Geometry check sheet. Reference: the model listing, model coordinates, mm. Face numbers are marked on the shaded views. Coordinates: 2 decimals unless noted, no trailing zeros. Write each loop counter-clockwise with the first axis right and the second up, starting at its lowest first coordinate (ties: lowest second). Pieces come first, ordered by that corner, then holes. Notation, with made-up numbers: (19.25, 1.25) -> (47.25, 1.25) arc R6 ccw to (47.25, 7.25) -> close; hole circle Ø8 at (36, -28). An arc over 180 degrees is marked (long way). Answer in a Markdown table with one row per item. Add a question column.
Q1. Section check C-C, the plane y = 44.5. Record the boundary of the cut face in (x, z), and give its area (3 significant figures).
Q2. Gauge pin test, flat ends, axial feed: P1, Ø5, axis at y = -13, z = 12, coming from the +X side; P2, Ø1, axis at x = -21, z = 4, coming from the +Y side; P3, Ø6, axis at x = -25.5, z = 15.5, coming from the +Y side. Record the tip position at first contact, or that the pin passes through.
Q3. Section check B-B, the plane x = 42. Record the boundary of the cut face in (y, z), and give its area (3 significant figures).
Q4. Section check A-A, the plane z = 11.25. Record the boundary of the cut face in (x, y).
Q5. Thickness scan on line 1 (Y direction, x = 1.5, z = 6); line 2 (Y direction, x = -4.5, z = 16.6); line 3 (X direction, y = -4.5, z = 15.85). Record the ranges inside material, lowest first.
Q6. Section check D-D, the plane x = -7.5. Count the separate pieces of the cut face and the enclosed holes in it, and give its area (3 significant figures).
Q7. Release check for a two-part mould opening along X. For the marked faces 1, 2 and 3 record: pulls with the +X half, pulls with the -X half, needs draft (parallel to the pull), parting line crosses it, or undercut.
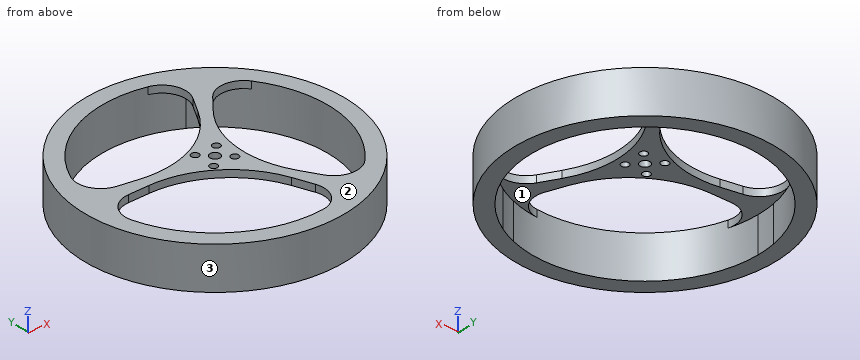
```python
from build123d import *

# Parameters (mm, degrees)
ESQUISSE1_R             = 55
BOSS_EXTRU_1_DEPTH      = 18
ESQUISSE2_R             = 2.1
ENL_V_MAT_EXTRU_1_DEPTH = 80.837334625
ENL_V_MAT_EXTRU_2_DEPTH = 80.837334625
ENL_V_MAT_EXTRU_3_DEPTH = 80.837334625
ENL_V_START             = 15
ESQUISSE8_R             = 48
ENL_V_MAT_EXTRU_4_DEPTH = 15
CONG_3_R                = 10
CONG_4_R                = 10
CONG_5_R                = 60
CONG_7_R                = 40
ESQUISSE10_R            = 1.6
ENL_V_MAT_EXTRU_9_DEPTH = 80.837334785


with BuildPart() as part:
    # Esquisse1 → Boss.-Extru.1 (new body)
    with BuildSketch(Plane.XY):
        Circle(ESQUISSE1_R)
    extrude(amount=BOSS_EXTRU_1_DEPTH)

    # Esquisse2 → Enlèv. mat.-Extru.1 (cut, through all)
    with BuildSketch(Plane.XY.offset(18)):
        Circle(ESQUISSE2_R)
    extrude(amount=-ENL_V_MAT_EXTRU_1_DEPTH, mode=Mode.SUBTRACT)

    # Esquisse3 → Enlèv. mat.-Extru.2 (cut, through all)
    with BuildSketch(Plane.XY.offset(18)):
        with BuildLine():
            ThreePointArc((-7.5, 0), (-4.301823273, -6.143640332), (2.565151075, -7.047694656))
            Line((2.565151075, -7.047694656), (16.41696688, -45.105245798))
            ThreePointArc((16.41696688, -45.105245798), (-27.531668945, -39.319298126), (-48, 0))
            Line((-48, 0), (-7.5, 0))
        make_face()
        with BuildLine():
            ThreePointArc((-47.270772145, 8.335112528), (-20.285676564, 43.502773778), (24, 41.569219382))
            Line((24, 41.569219382), (3.75, 6.495190528))
            ThreePointArc((3.75, 6.495190528), (-3.169636963, 6.797308403), (-7.386058148, 1.302361333))
            Line((-7.386058148, 1.302361333), (-47.270772145, 8.335112528))
        make_face()
        with BuildLine():
            ThreePointArc((30.853805265, 36.77013327), (47.817345508, -4.183475652), (24, -41.569219382))
            Line((24, -41.569219382), (3.75, -6.495190528))
            ThreePointArc((3.75, -6.495190528), (7.471460236, -0.653668071), (4.820907073, 5.745333323))
            Line((4.820907073, 5.745333323), (30.853805265, 36.77013327))
        make_face()
    extrude(amount=-ENL_V_MAT_EXTRU_2_DEPTH, mode=Mode.SUBTRACT)

    # Esquisse7 → Enlèv. mat.-Extru.3 (cut, through all)
    with BuildSketch(Plane.XY):
        with BuildLine():
            Line((2.565151075, -7.047694656), (-27.531668945, -39.319298126))
            Line((-27.531668945, -39.319298126), (-7.5, 0))
            ThreePointArc((-7.5, 0), (-3.331557771, -4.75795759), (2.565151075, -7.047694656))
        make_face()
        with BuildLine():
            Line((4.820907073, 5.745333323), (47.817345508, -4.183475652))
            Line((47.817345508, -4.183475652), (3.75, -6.495190528))
            ThreePointArc((3.75, -6.495190528), (5.786291029, -0.506234869), (4.820907073, 5.745333323))
        make_face()
        with BuildLine():
            Line((3.75, 6.495190528), (-20.285676564, 43.502773778))
            Line((-20.285676564, 43.502773778), (-7.386058148, 1.302361333))
            ThreePointArc((-7.386058148, 1.302361333), (-2.454733258, 5.264192459), (3.75, 6.495190528))
        make_face()
    extrude(amount=ENL_V_MAT_EXTRU_3_DEPTH, mode=Mode.SUBTRACT)

    # Esquisse8 → Enlèv. mat.-Extru.4 (cut)
    with BuildSketch(Plane.XY.offset(ENL_V_START)):
        Circle(ESQUISSE8_R)
    extrude(amount=-ENL_V_MAT_EXTRU_4_DEPTH, mode=Mode.SUBTRACT)

    # Congé3
    # the kernel refuses this fillet: 10 mm, written as the material it adds along each edge
    with BuildSketch(Plane(origin=(-47.270772145, 8.335112528, 18), x_dir=(0.3028483404391726, 0.9530387624295452, 0), z_dir=(0, 0, -1))) as cong_3_piece_1:
        with BuildLine():
            CenterArc((11.416839641, 9.911490246), CONG_3_R, 172.371238355, 105.25752329)
            Line((1.505349395, 11.239029739), (0, 0))
            ThreePointArc((0, 0), (6.372189567, -0.42484682), (12.744379134, 0))
        make_face()
    extrude(amount=3)
    with BuildSketch(Plane(origin=(24, 41.569219382, 18), x_dir=(-0.9247372088845717, 0.38060621973947306, 0), z_dir=(0, 0, -1)), Plane(origin=(24, -41.569219382, 18), x_dir=(0.7919832595750325, 0.6105428048490187, 0), z_dir=(0, 0, -1)), Plane(origin=(-48, 0, 18), x_dir=(0.13275394930954024, -0.9911490245884924, 0), z_dir=(0, 0, -1))) as cong_3_piece_2:
        with BuildLine():
            CenterArc((11.416839641, -9.911490246), CONG_3_R, 82.371238355, 105.25752329)
            Line((1.505349395, -11.239029739), (0, 0))
            ThreePointArc((0, 0), (6.372189567, 0.42484682), (12.744379134, 0))
        make_face()
    extrude(amount=3)
    with BuildSketch(Plane(origin=(16.41696688, -45.105245798, 18), x_dir=(-0.34202014332566844, 0.9396926207859085, 0), z_dir=(0, 0, -1))) as cong_3_piece_3:
        with BuildLine():
            CenterArc((11.33939444, -10), CONG_3_R, 90, 105.25752329)
            ThreePointArc((1.691866661, -12.631578947), (0.42484682, -6.372189567), (0, 0))
            Line((0, 0), (11.33939444, 0))
        make_face()
    extrude(amount=3)

    # Congé4
    # the kernel refuses this fillet: 10 mm, written as the material it adds along each edge
    with BuildSketch(Plane(origin=(30.853805265, 36.77013327, 18), x_dir=(0.6739316088356829, -0.7387937375290534, 0), z_dir=(0, 0, -1))) as cong_4_piece_1:
        with BuildLine():
            CenterArc((11.416839641, 9.911490246), CONG_4_R, 172.371238355, 105.25752329)
            Line((1.505349395, 11.239029739), (0, 0))
            ThreePointArc((0, 0), (6.372189567, -0.42484682), (12.744379134, 0))
        make_face()
    extrude(amount=3)

    # Congé5
    # the kernel refuses this fillet: 60 mm, written as the material it adds along each edge
    with BuildSketch(Plane(origin=(-7.386058148, 1.302361333, 18), x_dir=(0.8285733508252506, 0.5598805250249523, 0), z_dir=(0, 0, -1)), Plane(origin=(2.565151075, -7.047694656, 18), x_dir=(-0.8991574331684032, 0.4376253082009868, 0), z_dir=(0, 0, -1))) as cong_5_piece_1:
        with BuildLine():
            CenterArc((27.479152806, -56.896321194), CONG_5_R, 108.509321534, 25.538214121)
            Line((-14.236143248, -13.770527577), (0, 0))
            ThreePointArc((0, 0), (4.215808312, -0.686940021), (8.431616624, 0))
        make_face()
    extrude(amount=3)
    with BuildSketch(Plane(origin=(3.75, 6.495190528, 18), x_dir=(0.4999999999999999, 0.8660254037844387, 0), z_dir=(0, 0, -1)), Plane(origin=(-7.5, 0, 18), x_dir=(-1, 0, 0), z_dir=(0, 0, -1))) as cong_5_piece_2:
        with BuildLine():
            CenterArc((19.806443505, -60), CONG_5_R, 90, 25.538214121)
            ThreePointArc((-6.060335973, -5.862123061), (-2.552569547, -3.424808757), (0, 0))
            Line((0, 0), (19.806443505, 0))
        make_face()
    extrude(amount=3)
    with BuildSketch(Plane(origin=(4.820907073, 5.745333323, 18), x_dir=(0.6427876096865399, 0.7660444431189776, 0), z_dir=(0, 0, -1))) as cong_5_piece_3:
        with BuildLine():
            CenterArc((19.806443505, 60), CONG_5_R, 244.461785879, 25.538214121)
            ThreePointArc((-6.060335973, 5.862123061), (-2.552569547, 3.424808757), (0, 0))
            Line((0, 0), (19.806443505, 0))
        make_face()
    extrude(amount=3)
    with BuildSketch(Plane(origin=(3.75, -6.495190528, 18), x_dir=(0.24272682168261056, 0.9700946809646254, 0), z_dir=(0, 0, -1))) as cong_5_piece_4:
        with BuildLine():
            CenterArc((27.479152806, 56.896321194), CONG_5_R, 225.952464345, 25.538214121)
            Line((-14.236143248, 13.770527577), (0, 0))
            ThreePointArc((0, 0), (4.215808312, 0.686940021), (8.431616624, 0))
        make_face()
    extrude(amount=3)

    # Congé7
    cong_7_edges = [part.edges().sort_by_distance(p)[0] for p in [
        (-2.549741992, 5.467939348, 16.5),
        (6.010245378, -0.525828336, 16.5),
        (-3.460503385, -4.942111012, 16.5),
    ]]
    fillet(cong_7_edges, radius=CONG_7_R)

    # Esquisse10 → Enlèv. mat.-Extru.9 (cut, through all)
    with BuildSketch(Plane.XY):
        with Locations((-4.5, -4.5)):
            Circle(ESQUISSE10_R)
        with Locations((-4.5, 4.5)):
            Circle(ESQUISSE10_R)
        with Locations((4.5, 4.5)):
            Circle(ESQUISSE10_R)
        with Locations((4.5, -4.5)):
            Circle(ESQUISSE10_R)
    extrude(amount=ENL_V_MAT_EXTRU_9_DEPTH, mode=Mode.SUBTRACT)


solid = part.part
```
Calculated:
| question | item | result |
|---|---|---|
| 1 | outline | (-32.32, 0) -> (-17.99, 0) -> (-17.99, 18) -> (-32.32, 18) -> close; (15.99, 15) -> (17.99, 15) -> (17.99, 0) -> (32.32, 0) -> (32.32, 18) -> (15.99, 18) -> close |
| 1 | area | 522 mm² |
| 2 | P1 | stops at x = 53.99 |
| 2 | P2 | stops at y = 51.04 |
| 2 | P3 | stops at y = 50.19 |
| 3 | outline | (-35.51, 0) -> (-23.24, 0) -> (-23.24, 18) -> (-35.51, 18) -> close; (23.24, 0) -> (35.51, 0) -> (35.51, 18) -> (23.24, 18) -> close |
| 3 | area | 442 mm² |
| 4 | outline | circle Ø110 at (0, 0); hole circle Ø96 at (0, 0) |
| 5 | line 1 | y = -54.98 to -47.98, 47.98 to 54.98 |
| 5 | line 2 | y = -54.82 to -47.79, -7.64 to -6.1, -2.9 to 2.9, 6.1 to 7.66, 47.79 to 54.82 |
| 5 | line 3 | x = -54.82 to -45.01, -9.58 to -6.1, -2.9 to 2.9, 6.1 to 8.65, 47.79 to 54.82 |
| 6 | separate pieces | 3 |
| 6 | enclosed holes | 0 |
| 6 | area | 291 mm² |
| 7 | face 1 | undercut |
| 7 | face 2 | needs draft |
| 7 | face 3 | parting line crosses it |
